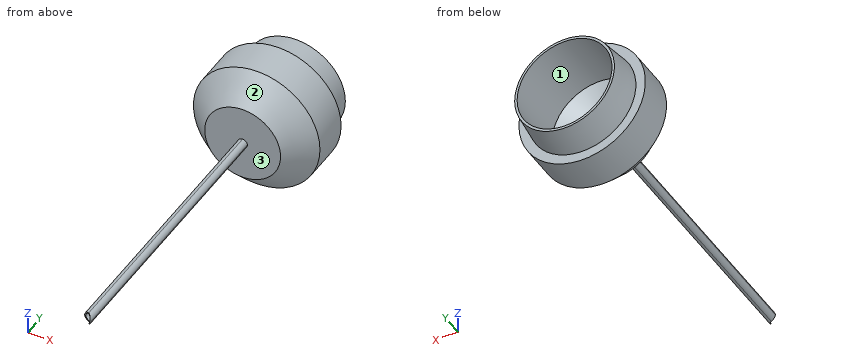
```python
from build123d import *

# Parameters (mm, degrees)
F0_R      = 21.59
F1_DEPTH  = 12.7
F2_R      = 25.4
F3_DEPTH  = 25.4
F4_SIZE   = 10.16
F5_W      = 3.81
F5_H      = 3.81
F6_DEPTH  = 114.3
F8_D      = 7.62
F9_R      = 1.9049
F11_D     = 38.1
F11_DEPTH = 25.4
F11_TIP   = 11.4463947925
F13_D     = 2.921
F13_DEPTH = 254
F13_START = 35.9688379
F13_TIP   = 0.8775569341
F14_SIZE2 = 1.559354
F14_SIZE  = 12.69999


# Not quite as in the source:
# - a fillet or chamfer is up to 0.001 mm smaller than in the source, because OpenCascade refuses the exact size


with BuildPart() as f1:
    # F0 (on Front) → F1 (new body)
    with BuildSketch(Plane.XZ):
        Circle(F0_R)
    extrude(amount=F1_DEPTH)

    # F2 (on face) → F3 (join)
    with BuildSketch(Plane.XZ.offset(12.7)):
        Circle(F2_R)
    extrude(amount=F3_DEPTH)

    # F4
    f4_edges = [f1.edges().sort_by_distance(p)[0] for p in [
        (-25.4, -38.1, 0),
    ]]
    chamfer(f4_edges, length=F4_SIZE)

    # F5 (on face) → F6 (join)
    with BuildSketch(Plane.XZ.offset(38.1)):
        Rectangle(F5_W, F5_H)
    extrude(amount=F6_DEPTH)

    # F8 (through all)
    with Locations(Plane.XY.offset(1.905)):
        with Locations((-1.905, -152.4)):
            Hole(F8_D / 2)

    # F9 (radius 1.905 in the source; OpenCascade refuses exactly that, so slightly less here)
    f9_edges = [f1.edges().sort_by_distance(p)[0] for p in [
        (1.905, -95.25, -1.905),
        (1.905, -95.25, 1.905),
        (-1.905, -93.345, 1.905),
        (-1.905, -93.345, -1.905),
    ]]
    fillet(f9_edges, radius=F9_R)

    # F11
    with Locations(Plane(origin=(0, 0, 0), x_dir=(-1, 0, 0), z_dir=(0, 1, 0))):
        with Locations((0, 0)):
            Hole(F11_D / 2, depth=F11_DEPTH)
            with Locations((0, 0, -(F11_DEPTH + F11_TIP / 2))):  # 118° drill point
                Cone(0, F11_D / 2, F11_TIP, mode=Mode.SUBTRACT)

    # F13
    # its depths count from where the whole tool has entered the part; down to there all is cleared
    with Locations(Plane(origin=(0, 0, 0), x_dir=(1, 0, 0), z_dir=(0, 1, 0)).offset(-F13_START)):
        with Locations((0, 0)):
            Hole(F13_D / 2, depth=F13_DEPTH)
            with Locations((0, 0, -(F13_DEPTH + F13_TIP / 2))):  # 118° drill point
                Cone(0, F13_D / 2, F13_TIP, mode=Mode.SUBTRACT)

    # F14 (size 12.7 and 1.5593639235 in the source; OpenCascade refuses exactly that, so slightly less here)
    f14_edges = [f1.edges().sort_by_distance(p)[0] for p in [
        (-21.59, 0, 0),
    ]]
    f14_side = f1.faces().sort_by_distance((-21.59, -6.35, 0))[0]
    chamfer(f14_edges, length=F14_SIZE, length2=F14_SIZE2, reference=f14_side)


solid = f1.part
```
Check sheet for the modelled part. Datum: model origin and axes. Units: mm. Face numbers are marked on the shaded views. Round coordinates to 2 decimals unless told otherwise and drop trailing zeros. One line per item, written item: value. Start each with the question number.
Q1. Mould release check, pull along X, two halves, no side actions. Record for the marked faces 1, 2 and 3: pulls with the +X half, pulls with the -X half, needs draft (parallel to the pull), parting line crosses it, or undercut.
Q2. Gauge pin test, flat ends, axial feed: pin 1 Ø5 at (y, z) = (-105.5, 1.5) entering from -X (3 decimals); pin 2 Ø3 at (y, z) = (-128, 4) entering from +X; pin 3 Ø2 at (y, z) = (-26.5, 17) entering from +X; pin 4 Ø3 at (x, z) = (-5, 17) entering from +Y. Record the tip position at first contact, or that the pin passes through.
Q3. Thickness scan on line 1 (X direction, y = -83.5, z = 0) (1 decimal); line 2 (Z direction, x = 0, y = -19.25); line 3 (Z direction, x = 0, y = -8.5). Record the ranges inside material, lowest first.
Completed:
1. face 1: undercut
1. face 2: parting line crosses it
1. face 3: needs draft
2. pin 1: stops at x = -1.905
2. pin 2: passes through
2. pin 3: stops at x = 19.73
2. pin 4: stops at y = 0
3. line 1: x = -1.9 to -1.5, 1.5 to 1.9
3. line 2: z = -25.4 to -19.05, 19.05 to 25.4
3. line 3: z = -21.07 to -19.05, 19.05 to 21.07
